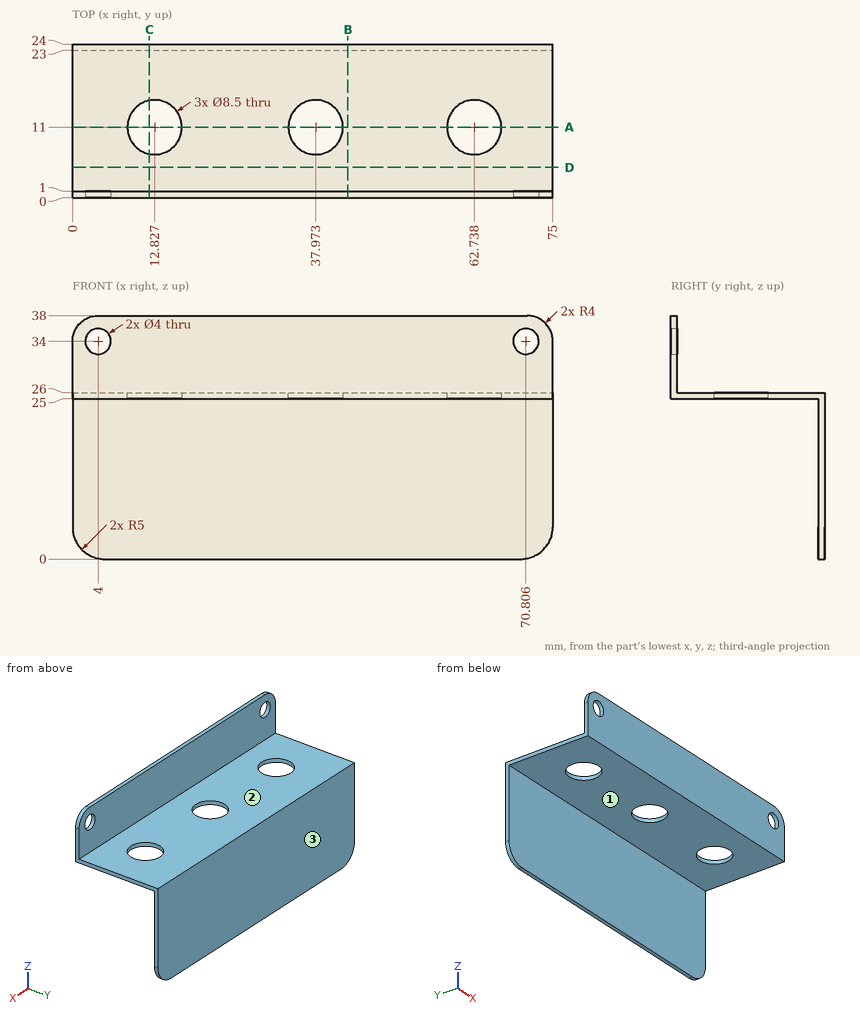
Geometry check sheet. Reference: drawing and pictorial views, mm from the part's lowest x, y, z. A direction names the side the tool comes from. Round coordinates to 2 decimals unless told otherwise and drop trailing zeros. Order: outer loops, then holes, each group sorted by start corner. A loop starts at its lowest first (then second) coordinate and runs counter-clockwise, first axis right, second up. Notation, with made-up numbers: M 3.5,88 L 52.5,88 A16 ccw 52.5,106 Z; hole C 51.25,31 d8. An arc over 180 degrees is marked long. One line per item, written item: value. Start each with the question number.
1. Section check B-B on x = 43. Enter the section's corners in (y, z), and give its area (3 significant figures).
2. Scan lines: line 1 along Z through (x, y) = (54.5, 17.25); line 2 along Y through (x, z) = (9, 31.5); line 3 along Y through (x, z) = (9.5, 7.5). Record each from-to range of solid material in increasing order.
3. Section check A-A on y = 11. Enter the section's corners in (x, z), and give its area (3 significant figures).
4. Section check D-D on y = 4.75. Enter the section's corners in (x, z), and give its area (3 significant figures).
5. Gauge pin test, flat ends, axial feed: P1, Ø7.5, axis at x = 52.5, z = 6.5, coming from the -Y side; P2, Ø3.5, axis at x = 4, z = 34, coming from the +Y side; P3, Ø5, axis at x = 63, y = 8, coming from the -Z side; P4, Ø6, axis at x = 56.5, y = 8.5, coming from the +Z side. Record the tip position at first contact, or that the pin passes through.
6. Access from +Z, -Z, +X, -X, +Y, -Y to the whole of each face (thin tool, end or side, straight path). Record for the marked faces 1, 2 and 3.
7. Section check C-C on x = 12. Enter the section's corners in (y, z).
Results found:
1. outline: M 0,25 L 23,25 L 23,0 L 24,0 L 24,26 L 1,26 L 1,38 L 0,38 Z
1. area: 61.0 mm^2
2. line 1: 25 to 26
2. line 2: 0 to 1
2. line 3: 23 to 24
3. outline: M 0,25 L 8.58,25 L 8.58,26 L 0,26 Z; M 17.08,25 L 33.72,25 L 33.72,26 L 17.08,26 Z; M 42.22,25 L 58.49,25 L 58.49,26 L 42.22,26 Z; M 66.99,25 L 75,25 L 75,26 L 66.99,26 Z
3. area: 49.5 mm^2
4. outline: M 0,25 L 75,25 L 75,26 L 0,26 Z
4. area: 75.0 mm^2
5. P1: y = 23
5. P2: through
5. P3: z = 25
5. P4: z = 26
6. face 1: -Z, +X, -X, -Y
6. face 2: +Z, +X, -X, +Y
6. face 3: +Z, -Z, +X, -X, +Y
7. outline: M 0,25 L 6.83,25 L 6.83,26 L 1,26 L 1,38 L 0,38 Z; M 15.17,25 L 23,25 L 23,0 L 24,0 L 24,26 L 15.17,26 Z
